For this review, take the finished solid that the model builds, in its own axes (mm). Round coordinates to 2 decimals unless told otherwise and drop trailing zeros. Write each loop counter-clockwise with the first axis right and the second up, starting at its lowest first coordinate (ties: lowest second). Pieces come first, ordered by that corner, then holes. Notation, with made-up numbers: (-34, 11) - (-20, 11) arc R13 cw to (-20, 16) - close; hole circle Ø8 at (6.5, -24.75). An arc over 180 degrees is marked (long way). Answer in a Markdown table with one row per item. Add a question column.
from build123d import *

# Parameters (mm, degrees)
ESQUISSE1_R             = 2.05
ESQUISSE1_R_2           = 3.2
BOSS_EXTRU_1_DEPTH      = 5
ESQUISSE2_W             = 90
ESQUISSE2_H             = 2
ENL_V_MAT_EXTRU_1_DEPTH = 69.080834307
CONG_1_R                = 1


with BuildPart() as part:
    # Esquisse1 → Boss.-Extru.1 (new body)
    with BuildSketch(Plane(origin=(0, 0, 0), x_dir=(1, 0, 0), z_dir=(0, 1, 0))):
        with BuildLine():
            Line((-66, 0), (66, 0))
            ThreePointArc((66, 0), (66.707106781, 0.292893219), (67, 1))
            Line((67, 1), (67, 10))
            ThreePointArc((67, 10), (66.707106781, 10.707106781), (66, 11))
            Line((66, 11), (-66, 11))
            ThreePointArc((-66, 11), (-66.707106781, 10.707106781), (-67, 10))
            Line((-67, 10), (-67, 1))
            ThreePointArc((-67, 1), (-66.707106781, 0.292893219), (-66, 0))
        make_face()
        with Locations(Location((60, 5.5, 0), (0, 0, 270))):
            Circle(ESQUISSE1_R, mode=Mode.SUBTRACT)
        with Locations(Location((33.5, 5.5, 0), (0, 0, 270))):
            Circle(ESQUISSE1_R_2, mode=Mode.SUBTRACT)
        with Locations(Location((-33.5, 5.5, 0), (0, 0, 90))):
            Circle(ESQUISSE1_R_2, mode=Mode.SUBTRACT)
        with Locations(Location((-60, 5.5, 0), (0, 0, 90))):
            Circle(ESQUISSE1_R, mode=Mode.SUBTRACT)
    extrude(amount=BOSS_EXTRU_1_DEPTH)

    # Esquisse2 → Enlèv. mat.-Extru.1 (cut, through all)
    with BuildSketch(Plane.XY):
        with Locations((0, 4)):
            Rectangle(ESQUISSE2_W, ESQUISSE2_H)
    extrude(amount=-ENL_V_MAT_EXTRU_1_DEPTH, mode=Mode.SUBTRACT)

    # Congé1
    cong_1_edges = [part.edges().sort_by_distance(p)[0] for p in [
        (-45, 4, -11),
        (45, 4, 0),
        (0, 3, -11),
        (45, 4, -11),
        (-45, 4, 0),
        (0, 3, 0),
    ]]
    fillet(cong_1_edges, radius=CONG_1_R)


solid = part.part
Q1. Add section B-B on y = 4.1. State the section outline as (x, z) points.
Q2. Insertion check: pin 1 Ø3 at (x, y) = (-3.5, 4) entering from -Z. The pin has a flat end and moves straight along its axis. Give the tip position at first contact, or say it passes through.
Q3. To check wall thickness, follow probe 1 along X at (y, z) = (1.25, -5.5); probe 2 along Z at (x, y) = (-60, 2.8); probe 3 along X at (y, z) = (3.3, -5.5). State the ranges of each line that lie inside material, in increasing order.
Q4. Add section D-D on x = 25.5. State the section outline as (y, z) points, then the cut area to 3 significant figures.
Q5. Add section A-A on z = -5.5. State the section outline as (x, y) points.
Q6. Draft analysis for pull direction Z (two halves, no side actions). For faces 1 (the face through (-1, 3, -5)), 2 (the face through (-36.673, 1.479, -5.083)), 3 (the face through (1, 1, -11)), state which applies: released by +Z, released by -Z, zero draft, split by the parting line, or undercut.
Q7. Add section C-C on x = 60. State the section outline as (y, z) points.
Answer sheet:
| question | item | result |
|---|---|---|
| 1 | outline | (-67, -10) arc R1 ccw to (-66, -11) - (-46, -11) arc R1 ccw to (-45, -10) - (-45, -1) arc R1 ccw to (-46, 0) - (-66, 0) arc R1 ccw to (-67, -1) - close; (45, -10) arc R1 ccw to (46, -11) - (66, -11) arc R1 ccw to (67, -10) - (67, -1) arc R1 ccw to (66, 0) - (46, 0) arc R1 ccw to (45, -1) - close; hole circle Ø4.1 at (-60, -5.5); hole circle Ø4.1 at (60, -5.5) |
| 2 | pin 1 | stops at z = -10.87 |
| 3 | probe 1 | x = -67 to -62.05, -57.95 to -36.7, -30.3 to 30.3, 36.7 to 57.95, 62.05 to 67 |
| 3 | probe 2 | z = -11 to -7.55, -3.45 to 0 |
| 3 | probe 3 | x = -67 to -62.05, -57.95 to -45, 45 to 57.95, 62.05 to 67 |
| 4 | outline | (0, -11) - (2, -11) arc R1 ccw to (3, -10) - (3, -1) arc R1 ccw to (2, 0) - (0, 0) - close |
| 4 | area | 32.6 mm² |
| 5 | outline | (-67, 0) - (-62.05, 0) - (-62.05, 5) - (-67, 5) - close; (-57.95, 0) - (-36.7, 0) - (-36.7, 3) - (-45, 3) - (-45, 5) - (-57.95, 5) - close; (-30.3, 0) - (30.3, 0) - (30.3, 3) - (-30.3, 3) - close; (36.7, 0) - (57.95, 0) - (57.95, 5) - (45, 5) - (45, 3) - (36.7, 3) - close; (62.05, 0) - (67, 0) - (67, 5) - (62.05, 5) - close |
| 6 | face 1 | zero draft |
| 6 | face 2 | undercut |
| 6 | face 3 | released by -Z |
| 7 | outline | (0, -11) - (5, -11) - (5, -7.55) - (0, -7.55) - close; (0, -3.45) - (5, -3.45) - (5, 0) - (0, 0) - close |
